CAD build for the part. Positions are in the model's coordinates, mm. Face numbers are marked on the shaded views. A direction names the side the tool comes from. Coordinates: 2 decimals unless noted, no trailing zeros. Loops run counter-clockwise (first coordinate to the right, second up) from the corner with the lowest first, then second, coordinate; pieces in that order, holes last. Notation, with made-up numbers: (9.5, 28) - (56.5, 28) arc R24 ccw to (56.5, 65) - close; hole circle Ø5 at (14, 83.25). An arc over 180 degrees is marked (long way). Put each result on its own line as item: value.
```python
from build123d import *

# Parameters (mm, degrees)
SKETCH1_W           = 40
SKETCH1_H           = 40
BOSS_EXTRUDE1_DEPTH = 17
SKETCH2_R           = 5
BOSS_EXTRUDE2_DEPTH = 10


with BuildPart() as part:
    # Sketch1 → Boss-Extrude1 (new body)
    with BuildSketch(Plane(origin=(0, 0, 0), x_dir=(1, 0, 0), z_dir=(0, 1, 0))):
        Rectangle(SKETCH1_W, SKETCH1_H)
    extrude(amount=BOSS_EXTRUDE1_DEPTH)

    # Sketch2 → Boss-Extrude2 (add)
    with BuildSketch(Plane(origin=(0, 0, -20), x_dir=(-1, 0, 0), z_dir=(0, 0, -1))):
        with Locations((10, 5)):
            Circle(SKETCH2_R)
    boss_extrude2 = extrude(amount=BOSS_EXTRUDE2_DEPTH)

    # Mirror1: Boss-Extrude2 across plane
    add(boss_extrude2.mirror(Plane(origin=(0, 0, 0), x_dir=(0, 0, 1), z_dir=(1, 0, 0))))


solid = part.part
```
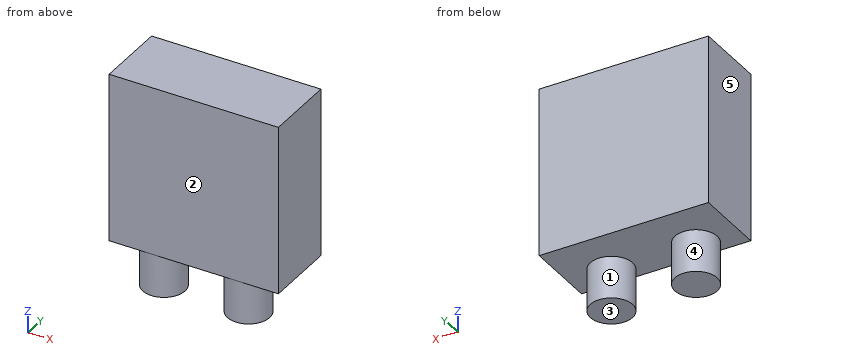
Q1. Slice it at A-A, the plane x = -13. Give the cut face in (y, z), then the cut area to 3 significant figures.
Determined:
outline: (0, -20) - (1, -20) - (1, -30) - (9, -30) - (9, -20) - (17, -20) - (17, 20) - (0, 20) - close
area: 760 mm2
Q2. Slice it at C-C, the plane z = -26. Give the cut face in (x, y), then the cut area to 3 significant figures.
Determined:
outline: circle Ø10 at (-10, 5); circle Ø10 at (10, 5)
area: 157 mm2
Q3. Wall check: L1, parallel to Z at x = -3, y = 10.25; L2, parallel to X at y = 4, z = -21.5; L3, parallel to Y at x = -9, z = -21. Give the ranges that are in metal, low to high. Write a range as from..to.
Determined:
L1: -20..20
L2: -14.9..-5.1, 5.1..14.9
L3: 0.1..9.9
Q4. Slice it at B-B, the plane y = 8. Give the cut face in (x, z).
Determined:
outline: (-20, -20) - (-14, -20) - (-14, -30) - (-6, -30) - (-6, -20) - (6, -20) - (6, -30) - (14, -30) - (14, -20) - (20, -20) - (20, 20) - (-20, 20) - close
Q5. Pin check, flat tip, straight feed: pin 1 Ø12 at (x, z) = (13, -18.5) entering from -Y. Stop position of the tip, or through.
Determined:
pin 1: y = 0
Q6. Mould opens along X. For the marked faces 3, 4 and 5 say: +X half, -X half, draft (parallel to the pull), parting line (faces both ways), or undercut.
Determined:
face 3: draft
face 4: undercut
face 5: -X half
Q7. Slice it at D-D, the plane y = 1.75. Give the cut face in (x, z), then the cut area to 3 significant figures.
Determined:
outline: (-20, -20) - (-13.8, -20) - (-13.8, -30) - (-6.2, -30) - (-6.2, -20) - (6.2, -20) - (6.2, -30) - (13.8, -30) - (13.8, -20) - (20, -20) - (20, 20) - (-20, 20) - close
area: 1,750 mm2
Q8. Tool access for the marked faces 1 and 2: list every direction of +Z, -Z, +X, -X, +Y, -Y with a clear straight run to the whole face (end or side of a thin tool).
Determined:
face 1: -Z
face 2: +Z, -Z, +X, -X, -Y
